Source: CAD feature listing. Evaluate the final solid. Frame: model axes, mm. Face numbers are marked on the shaded views. A direction names the side the tool comes from. Give positions to 0.01 mm unless a question says otherwise; leave off trailing zeros. Write each loop counter-clockwise with the first axis right and the second up, starting at its lowest first coordinate (ties: lowest second). Pieces come first, ordered by that corner, then holes. Notation, with made-up numbers: M -29.5,24 L -24.5,24 A14 cw -24.5,38 Z; hole C -34,16 d10. An arc over 180 degrees is marked long. Use CSV: the item, a comma, the result in double quotes. Start each with the question number.
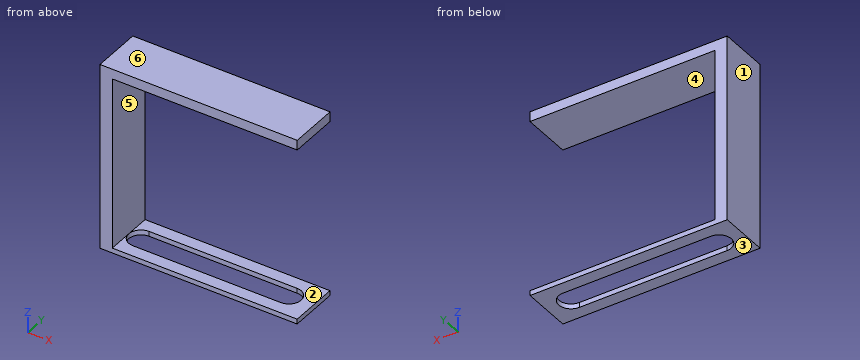
Autodesk Inventor part; units mm, degrees
ref_plane "YZ Plane" through (0, 0, 0) normal (1, 0, 0) x (0, 1, 0)
ref_plane "XZ Plane" through (0, 0, 0) normal (0, 1, 0) x (-1, 0, 0)
ref_plane "XY Plane" through (0, 0, 0) normal (0, 0, 1) x (1, 0, 0)
sketch "Esboço1" plane through (0, 0, 0) normal (0, 0, 1) x (1, 0, 0)
  line L0 (0, 0) -> (40, 0)
  line L1 (40, 0) -> (40, 10)
  line L2 (40, 10) -> (0, 10)
  line L3 (0, 10) -> (0, 0)
  dimension "d0" = 40
  dimension "d1" = 10
extrude "Extrusão1" add sketch "Esboço1" along normal blind 1
sketch "Esboço2" plane through (0, 0, 1) normal (0, 0, 1) x (1, 0, 0)
  line L0 (5, 5) -> (35, 5) construction
  line L1 (5, 2.5) -> (35, 2.5)
  line L2 (35, 7.5) -> (5, 7.5)
  arc A0 (5, 7.5) -> (5, 2.5) centre (5, 5) ccw
  arc A1 (35, 2.5) -> (35, 7.5) centre (35, 5) ccw
  point P0 (0, 0)
  point P1 (20, 5)
  dimension "d4" = 30
  dimension "d5" = 5
extrude "Extrusão2" cut sketch "Esboço2" against normal blind 1
sketch "Esboço3" plane through (0, 0, 1) normal (0, 0, 1) x (1, 0, 0)
  line L0 (40, 10) -> (0, 10)
  line L1 (0, 0) -> (40, 0)
  line L2 (0, 10) -> (2.5, 10)
  line L3 (2.5, 10) -> (2.5, 0)
  line L4 (2.5, 0) -> (0, 0)
  line L5 (0, 0) -> (0, 10)
  dimension "d8" = 2.5
extrude "Extrusão3" add sketch "Esboço3" along normal blind 35
sketch "Esboço4" plane through (0, 0, 36) normal (0, 0, 1) x (1, 0, 0)
  line L0 (0, 10) -> (0, 0)
  line L1 (0, 10) -> (40.017, 10)
  line L2 (40.017, 10) -> (40.017, 0)
  line L3 (40.017, 0) -> (0, 0)
  line L4 (0, 0) -> (0, 10)
extrude "Extrusão4" add sketch "Esboço4" along normal blind 2
properties part number "Suporte prensas coletor"
1. Section A-A on x = 10. Return loops of the section in (y, z), then the cut area to 3 significant figures.
2. Line query: probe 1 along Z at (x, y) = (22, 9); probe 2 along X at (y, z) = (8.75, 8); probe 3 along Z at (x, y) = (27.5, 6.75). Output: solid intervals per line, ascending.
3. First-contact query: pin 1 (4 mm diameter, centred on y = 1, z = 5.5, fed in from -X); pin 2 (3 mm diameter, centred on y = 4, z = 11, fed in from +X); pin 3 (1.1 mm diameter, centred on y = 5.5, z = 0.5, fed in from +X). Flat tips, straight axial feed; report the tip coordinate or a pass-through.
4. Section C-C on y = 1.5. Return loops of the section in (x, z).
5. Access query for the marked faces 1 and 2. Directions: +Z, -Z, +X, -X, +Y, -Y. A direction counts if a zero-diameter tool reaches every point of the face in a straight line with its end or side. Return the directions, or none.
6. Section D-D on x = 4. Return loops of the section in (y, z).
7. Section B-B on y = 6.75. Return loops of the section in (x, z), then the cut area to 3 significant figures.
8. Pull-direction query (Z, two-part tool) for the marked faces 3, 4, 5 and 6; classes: released by +Z, released by -Z, zero draft, split by the parting line, or undercut.
Resolved:
1,outline,"M 0,0 L 2.5,0 L 2.5,1 L 0,1 Z; M 0,36 L 10,36 L 10,38 L 0,38 Z; M 7.5,0 L 10,0 L 10,1 L 7.5,1 Z"
1,area,"25.0 mm2"
2,probe 1,"z = 0 to 1, 36 to 38"
2,probe 2,"x = 0 to 2.5"
2,probe 3,"z = 36 to 38"
3,pin 1,"stops at x = 0"
3,pin 2,"stops at x = 2.5"
3,pin 3,"stops at x = 40"
4,outline,"M 0,0 L 40,0 L 40,1 L 2.5,1 L 2.5,36 L 40.02,36 L 40.02,38 L 0,38 Z"
5,face 1,"+Z, -Z, -X, +Y, -Y"
5,face 2,"+X, +Y, -Y"
6,outline,"M 0,0 L 2.71,0 L 2.71,1 L 0,1 Z; M 0,36 L 10,36 L 10,38 L 0,38 Z; M 7.29,0 L 10,0 L 10,1 L 7.29,1 Z"
7,outline,"M 0,0 L 3.21,0 L 3.21,1 L 2.5,1 L 2.5,36 L 40.02,36 L 40.02,38 L 0,38 Z; M 36.79,0 L 40,0 L 40,1 L 36.79,1 Z"
7,area,"174 mm2"
8,face 3,"released by -Z"
8,face 4,"undercut"
8,face 5,"undercut"
8,face 6,"released by +Z"
